from build123d import *

# Parameters (mm, degrees)
SKETCH1_R           = 3
BOSS_EXTRUDE1_DEPTH = 27
CUT_EXTRUDE4_START  = -0.1
CUT_EXTRUDE4_DEPTH  = 0.1
BOSS_EXTRUDE4_DEPTH = 12
BOSS_EXTRUDE5_START = 5
BOSS_EXTRUDE5_DEPTH = 5
SKETCH14_R          = 2.5
BOSS_EXTRUDE7_DEPTH = 4
SKETCH15_R          = 19
BOSS_EXTRUDE8_DEPTH = 2
BOSS_EXTRUDE9_START = 30
SKETCH16_R          = 3
BOSS_EXTRUDE9_DEPTH = 30
SKETCH17_W          = 6
SKETCH17_H          = 6
CUT_EXTRUDE5_DEPTH  = 20


with BuildPart() as part:
    # Sketch1 → Boss-Extrude1 (new body)
    with BuildSketch(Plane(origin=(0, 0, 0), x_dir=(0, 0, -1), z_dir=(1, 0, 0))):
        with BuildLine():
            Line((-18.5, 28), (18.5, 28))
            ThreePointArc((18.5, 28), (21.282485579, 21.282485579), (28, 18.5))
            Line((28, 18.5), (28, -18.5))
            ThreePointArc((28, -18.5), (21.282485579, -21.282485579), (18.5, -28))
            Line((18.5, -28), (-18.5, -28))
            ThreePointArc((-18.5, -28), (-21.282485579, -21.282485579), (-28, -18.5))
            Line((-28, -18.5), (-28, 18.5))
            ThreePointArc((-28, 18.5), (-21.282485579, 21.282485579), (-18.5, 28))
        make_face()
        Circle(SKETCH1_R, mode=Mode.SUBTRACT)
    extrude(amount=BOSS_EXTRUDE1_DEPTH)

    # Sketch6 → Cut-Extrude4 (cut)
    with BuildSketch(Plane(origin=(27, 0, 0), x_dir=(0, 0, -1), z_dir=(1, 0, 0)).offset(CUT_EXTRUDE4_START)):
        with BuildLine():
            Line((28, -18.5), (28, 18.5))
            ThreePointArc((28, 18.5), (21.282485579, 21.282485579), (18.5, 28))
            Line((18.5, 28), (-18.5, 28))
            ThreePointArc((-18.5, 28), (-21.282485579, 21.282485579), (-28, 18.5))
            Line((-28, 18.5), (-28, -18.5))
            ThreePointArc((-28, -18.5), (-21.282485579, -21.282485579), (-18.5, -28))
            Line((-18.5, -28), (18.5, -28))
            ThreePointArc((18.5, -28), (21.282485579, -21.282485579), (28, -18.5))
        make_face()
        with BuildLine():
            Line((18.302062075, 27.8), (-18.302062075, 27.8))
            ThreePointArc((-18.302062075, 27.8), (-21.141064222, 21.141064222), (-27.8, 18.302062075))
            Line((-27.8, 18.302062075), (-27.8, -18.302062075))
            ThreePointArc((-27.8, -18.302062075), (-21.141064222, -21.141064222), (-18.302062075, -27.8))
            Line((-18.302062075, -27.8), (18.302062075, -27.8))
            ThreePointArc((18.302062075, -27.8), (21.141064222, -21.141064222), (27.8, -18.302062075))
            Line((27.8, -18.302062075), (27.8, 18.302062075))
            ThreePointArc((27.8, 18.302062075), (21.141064222, 21.141064222), (18.302062075, 27.8))
        make_face(mode=Mode.SUBTRACT)
    extrude(amount=CUT_EXTRUDE4_DEPTH, mode=Mode.SUBTRACT)

    # Sketch10 → Boss-Extrude4 (add)
    with BuildSketch(Plane(origin=(27, 0, 0), x_dir=(0, 0, -1), z_dir=(1, 0, 0))):
        with BuildLine():
            Line((27.8, -18.302062075), (27.8, 18.302062075))
            ThreePointArc((27.8, 18.302062075), (21.141064222, 21.141064222), (18.302062075, 27.8))
            Line((18.302062075, 27.8), (-18.302062075, 27.8))
            ThreePointArc((-18.302062075, 27.8), (-21.141064222, 21.141064222), (-27.8, 18.302062075))
            Line((-27.8, 18.302062075), (-27.8, -18.302062075))
            ThreePointArc((-27.8, -18.302062075), (-21.141064222, -21.141064222), (-18.302062075, -27.8))
            Line((-18.302062075, -27.8), (18.302062075, -27.8))
            ThreePointArc((18.302062075, -27.8), (21.141064222, -21.141064222), (27.8, -18.302062075))
        make_face()
    extrude(amount=BOSS_EXTRUDE4_DEPTH)

    # Sketch12 → Boss-Extrude5 (add)
    with BuildSketch(Plane.ZY.offset(BOSS_EXTRUDE5_START)):
        with BuildLine():
            Line((-27.8, 18.302062075), (-27.8, -18.302062075))
            ThreePointArc((-27.8, -18.302062075), (-21.141064222, -21.141064222), (-18.302062075, -27.8))
            Line((-18.302062075, -27.8), (18.302062075, -27.8))
            ThreePointArc((18.302062075, -27.8), (21.141064222, -21.141064222), (27.8, -18.302062075))
            Line((27.8, -18.302062075), (27.8, 18.302062075))
            ThreePointArc((27.8, 18.302062075), (21.141064222, 21.141064222), (18.302062075, 27.8))
            Line((18.302062075, 27.8), (-18.302062075, 27.8))
            ThreePointArc((-18.302062075, 27.8), (-21.141064222, 21.141064222), (-27.8, 18.302062075))
        make_face()
    extrude(amount=-BOSS_EXTRUDE5_DEPTH)

    # Sketch14 → Boss-Extrude7 (add)
    with BuildSketch(Plane.ZY.offset(5)):
        with BuildLine():
            Line((-26, 28), (26, 28))
            ThreePointArc((26, 28), (27.414213562, 27.414213562), (28, 26))
            Line((28, 26), (28, -26))
            ThreePointArc((28, -26), (27.414213562, -27.414213562), (26, -28))
            Line((26, -28), (-26, -28))
            ThreePointArc((-26, -28), (-27.414213562, -27.414213562), (-28, -26))
            Line((-28, -26), (-28, 26))
            ThreePointArc((-28, 26), (-27.414213562, 27.414213562), (-26, 28))
        make_face()
        with Locations((-24, 24)):
            Circle(SKETCH14_R, mode=Mode.SUBTRACT)
        with Locations((24, 24)):
            Circle(SKETCH14_R, mode=Mode.SUBTRACT)
        with Locations((24, -24)):
            Circle(SKETCH14_R, mode=Mode.SUBTRACT)
        with Locations((-24, -24)):
            Circle(SKETCH14_R, mode=Mode.SUBTRACT)
    extrude(amount=BOSS_EXTRUDE7_DEPTH)

    # Sketch15 → Boss-Extrude8 (add)
    with BuildSketch(Plane.ZY.offset(9)):
        Circle(SKETCH15_R)
    extrude(amount=BOSS_EXTRUDE8_DEPTH)

    # Sketch16 → Boss-Extrude9 (add)
    with BuildSketch(Plane.ZY.offset(11).offset(BOSS_EXTRUDE9_START)):
        Circle(SKETCH16_R)
    extrude(amount=-BOSS_EXTRUDE9_DEPTH)

    # Sketch17 → Cut-Extrude5 (cut)
    with BuildSketch(Plane.ZY.offset(41)):
        with Locations((0, 5)):
            Rectangle(SKETCH17_W, SKETCH17_H)
    extrude(amount=-CUT_EXTRUDE5_DEPTH, mode=Mode.SUBTRACT)


solid = part.part
Can you work these out from the model? Positions are in its coordinate system, mm. A direction names the side the tool comes from. Give positions to 0.01 mm unless a question says otherwise; leave off trailing zeros. Order: outer loops, then holes, each group sorted by start corner. A loop starts at its lowest first (then second) coordinate and runs counter-clockwise, first axis right, second up. Notation, with made-up numbers: M 11.5,44 L 22.5,44 A18 cw 22.5,61 Z; hole C 62,-27.5 d7. An arc over 180 degrees is marked long. Use a Markdown table: item, result. Add a question column.
Item 1: For faces 3 (the flat face through (-3, 0, 27.8)), 4 (the cylindrical face through (-26.21, -2.662, 1.384)), 5 (the cylindrical face through (13.262, 21.209, 21.357)), 6 (the cylindrical face through (32.865, -21.068, 21.215)), which set-ups out of +Z, -Z, +X, -X, +Y, -Y let a thin tool reach every point of the face, with its end or its side?
Item 2: If I drill on L1, parallel to Y at x = -6, z = -24; L2, parallel to Y at x = 5, z = 0; L3, parallel to Z at x = 9, y = -2, over which ranges is the centre line in solid material (lowest first)? Write a range as [from, to].
Item 3: Suppose I cut it at D-D (y = 24). List the corners of the cut face in (x, z) for me.
Item 4: Suppose I cut it at A-A (y = 0). List the corners of the cut face in (x, z) for me, then the cut area to 3 significant figures.
Item 5: Suppose I cut it at B-B (x = 7.5). List the corners of the cut face in (y, z) for me, then the cut area to 3 significant figures.
Item 6: Will these pins go through, and if not, where does the flat tip stop? pin 1 (3.5 mm diameter, centred on x = 36, y = -8, fed in from -Z); pin 2 (2 mm diameter, centred on x = -27, z = 0, fed in from +Y); pin 3 (13.5 mm diameter, centred on x = 34.5, z = 0.5, fed in from +Y).
Item 7: We'd pull the mould along X, two halves only. Please class faces 1 (the flat face through (27, 0, 0)), 2 (the flat face through (-7, 0, 28)): +X half, -X half, draft (parallel to the pull), parting line (faces both ways), or undercut.
Answer sheet:
| question | item | result |
|---|---|---|
| 1 | face 3 | +Z, +Y, -Y |
| 1 | face 4 | -X |
| 1 | face 5 | +Z, +X, +Y |
| 1 | face 6 | +Z, +X, -Y |
| 2 | L1 | y = [-28, -26.5], [-21.5, 21.5], [26.5, 28] |
| 2 | L2 | y = [-28, -3], [3, 28] |
| 2 | L3 | z = [-28, -2.24], [2.24, 28] |
| 3 | outline | M -9,-28 L -5,-28 L -5,-26.5 L -9,-26.5 Z; M -9,-21.5 L -5,-21.5 L -5,-19.16 L 0,-19.16 L 0,-19.38 L 26.9,-19.38 L 26.9,-19.16 L 39,-19.16 L 39,19.16 L 26.9,19.16 L 26.9,19.38 L 0,19.38 L 0,19.16 L -5,19.16 L -5,21.5 L -9,21.5 Z; M -9,26.5 L -5,26.5 L -5,28 L -9,28 Z |
| 4 | outline | M -41,-3 L -11,-3 L -11,-19 L -9,-19 L -9,-28 L -5,-28 L -5,-27.8 L 0,-27.8 L 0,-28 L 26.9,-28 L 26.9,-27.8 L 39,-27.8 L 39,27.8 L 26.9,27.8 L 26.9,28 L 0,28 L 0,27.8 L -5,27.8 L -5,28 L -9,28 L -9,19 L -11,19 L -11,3 L -41,3 Z; hole M 0,-3 L 27,-3 L 27,3 L 0,3 Z |
| 4 | area | 2,780 mm² |
| 5 | outline | M -28,-18.5 A9.5 cw -18.5,-28 L 18.5,-28 A9.5 cw 28,-18.5 L 28,18.5 A9.5 cw 18.5,28 L -18.5,28 A9.5 cw -28,18.5 Z; hole C 0,0 d6 |
| 5 | area | 2,820 mm² |
| 6 | pin 1 | stops at z = -27.8 |
| 6 | pin 2 | stops at y = 2 |
| 6 | pin 3 | stops at y = 27.8 |
| 7 | face 1 | undercut |
| 7 | face 2 | draft |
